Verification items for the finished model (mm, model axes). Face numbers are marked on the shaded views. A direction names the side the tool comes from. Round coordinates to 2 decimals unless told otherwise and drop trailing zeros. Write each loop counter-clockwise with the first axis right and the second up, starting at its lowest first coordinate (ties: lowest second). Pieces come first, ordered by that corner, then holes. Notation, with made-up numbers: M 10,2.5 L 55,2.5 A28 cw 55,40.5 Z; hole C 88,79.25 d8. An arc over 180 degrees is marked long. Answer in a Markdown table with one row per item. Add a question column.
1. Draft check along Y on the marked faces 1, 2 and 3. Enter one of: pulls with the +Y half, pulls with the -Y half, needs draft (parallel to the pull), parting line crosses it, or undercut.
2. Sectioned sample at D-D on z = 5.25. Record the cut outline in (x, y).
3. Go/stop test with flat-tipped pins: pin 1 Ø1 at (x, y) = (-8.5, 9) entering from +Z; pin 2 Ø1.5 at (x, y) = (25.5, 8) entering from -Z. Record where each tip stops, or that it passes through.
4. Sectioned sample at A-A on z = -7.5. Record the cut outline in (x, y), plus the area to 3 significant figures.
5. Set-up check for the marked faces 4 and 5: record each of +Z, -Z, +X, -X, +Y, -Y from which the full face is reachable in a straight line by a thin tool's end or side.
6. Sectioned sample at C-C on y = 22.5. Record the cut outline in (x, z).
7. Material ranges on probe 1 along Y at (x, z) = (-61.06, 0.25); probe 2 along X at (y, z) = (20, -5.75); probe 3 along Y at (x, z) = (-15, 4.5), recorded low to high.
8. Sectioned sample at B-B on x = -61.06. Record the cut outline in (y, z), plus the area to 3 significant figures.
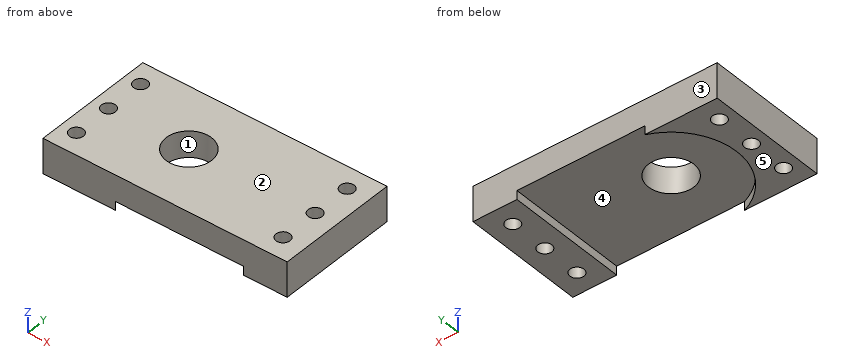
```python
from build123d import *

# Parameters (mm, degrees)
SKETCH1_W           = 140
SKETCH1_H           = 70
SKETCH1_R           = 13
SKETCH1_R_2         = 4
BOSS_EXTRUDE1_DEPTH = 10
CUT_EXTRUDE1_DEPTH  = 5


with BuildPart() as part:
    # Sketch1 → Boss-Extrude1 (new body, symmetric)
    with BuildSketch(Plane.XY):
        Rectangle(SKETCH1_W, SKETCH1_H)
        with Locations((-15, 0)):
            Circle(SKETCH1_R, mode=Mode.SUBTRACT)
        with Locations((57.4, 0)):
            Circle(SKETCH1_R_2, mode=Mode.SUBTRACT)
        with Locations((57.4, 22.5)):
            Circle(SKETCH1_R_2, mode=Mode.SUBTRACT)
        with Locations((-61.06, 0)):
            Circle(SKETCH1_R_2, mode=Mode.SUBTRACT)
        with Locations((-61.06, 22.5)):
            Circle(SKETCH1_R_2, mode=Mode.SUBTRACT)
        with Locations((-61.06, -22.5)):
            Circle(SKETCH1_R_2, mode=Mode.SUBTRACT)
        with Locations((57.4, -22.5)):
            Circle(SKETCH1_R_2, mode=Mode.SUBTRACT)
    extrude(amount=BOSS_EXTRUDE1_DEPTH, both=True)

    # Sketch2 → Cut-Extrude1 (cut)
    with BuildSketch(Plane(origin=(0, 0, -10), x_dir=(-1, 0, 0), z_dir=(0, 0, -1))):
        with BuildLine():
            Line((15, -37.5), (-44.8, -37.5))
            Line((-44.8, -37.5), (-44.8, 37.5))
            Line((-44.8, 37.5), (15, 37.5))
            ThreePointArc((15, 37.5), (52.5, 0), (15, -37.5))
        make_face()
    extrude(amount=-CUT_EXTRUDE1_DEPTH, mode=Mode.SUBTRACT)


solid = part.part
```
Geometry check:
| question | item | result |
|---|---|---|
| 1 | face 1 | undercut |
| 1 | face 2 | needs draft |
| 1 | face 3 | pulls with the +Y half |
| 2 | outline | M -70,-35 L 70,-35 L 70,35 L -70,35 Z; hole C -61.06,-22.5 d8; hole C -61.06,0 d8; hole C -61.06,22.5 d8; hole C -15,0 d26; hole C 57.4,-22.5 d8; hole C 57.4,0 d8; hole C 57.4,22.5 d8 |
| 3 | pin 1 | passes through |
| 3 | pin 2 | stops at z = -5 |
| 4 | outline | M -70,-35 L -28.46,-35 A37.5 cw -28.46,35 L -70,35 Z; M 44.8,-35 L 70,-35 L 70,35 L 44.8,35 Z; hole C -61.06,-22.5 d8; hole C -61.06,0 d8; hole C -61.06,22.5 d8; hole C 57.4,-22.5 d8; hole C 57.4,0 d8; hole C 57.4,22.5 d8 |
| 4 | area | 3,150 mm2 |
| 5 | face 4 | -Z |
| 5 | face 5 | -Z, +X, -X, +Y, -Y |
| 6 | outline | M -70,-10 L -65.06,-10 L -65.06,10 L -70,10 Z; M -57.06,-10 L -45,-10 L -45,-5 L 44.8,-5 L 44.8,-10 L 53.4,-10 L 53.4,10 L -57.06,10 Z; M 61.4,-10 L 70,-10 L 70,10 L 61.4,10 Z |
| 7 | probe 1 | y = -35 to -26.5, -18.5 to -4, 4 to 18.5, 26.5 to 35 |
| 7 | probe 2 | x = -70 to -64.18, -57.94 to -46.72, 44.8 to 54.28, 60.52 to 70 |
| 7 | probe 3 | y = -35 to -13, 13 to 35 |
| 8 | outline | M -35,-10 L -26.5,-10 L -26.5,10 L -35,10 Z; M -18.5,-10 L -4,-10 L -4,10 L -18.5,10 Z; M 4,-10 L 18.5,-10 L 18.5,10 L 4,10 Z; M 26.5,-10 L 35,-10 L 35,10 L 26.5,10 Z |
| 8 | area | 920 mm2 |
